Part model, mm, in its own coordinate system. Face numbers are marked on the shaded views. Give positions to 0.01 mm unless a question says otherwise; leave off trailing zeros. Order: outer loops, then holes, each group sorted by start corner. A loop starts at its lowest first (then second) coordinate and runs counter-clockwise, first axis right, second up. Notation, with made-up numbers: M 21,25 L 37,25 A13 ccw 37,49 Z; hole C -25.75,-4.5 d9. An arc over 180 degrees is marked long. Answer as a JSON object with one key per item and string values.
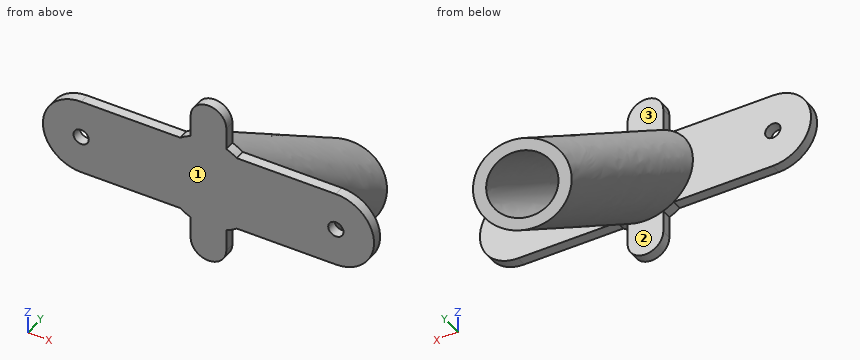
from build123d import *

# Parameters (mm, degrees)
CROQUIS1_R                 = 9.325
CROQUIS1_R_2               = 6.835
CROQUIS11_R                = 1.5
SALIENTE_EXTRUIR1_DEPTH    = 2
CORTAR_EXTRUIR2_DEPTH      = 69.96775808
CORTAR_EXTRUIR2_DEPTH_BACK = 69.96775808


with BuildPart() as part:
    # Barrer1: sweep along a path in Croquis6
    with BuildLine(Plane(origin=(0, 0, 0), x_dir=(0, 0, -1), z_dir=(1, 0, 0))) as barrer1_path:
        Line((9.345393917, 0), (40.892097916, 45.053362436))
    # Croquis1 → Barrer1 (sweep)
    with BuildSketch(Plane(origin=(0, 0, 0), x_dir=(1, 0, 0), z_dir=(0, 1, 0))):
        Circle(CROQUIS1_R)
        Circle(CROQUIS1_R_2, mode=Mode.SUBTRACT)
    sweep(path=barrer1_path.line)

    # Croquis11 → Saliente-Extruir1 (add)
    with BuildSketch(Plane.XZ):
        with BuildLine():
            Line((-25, 7.5), (-5.54126565, 7.5))
            ThreePointArc((-5.54126565, 7.5), (-4.556629397, 8.135892916), (-3.5, 8.643241579))
            Line((-3.5, 8.643241579), (-3.5, 13))
            ThreePointArc((-3.5, 13), (0, 16.5), (3.5, 13))
            Line((3.5, 13), (3.5, 8.643241579))
            ThreePointArc((3.5, 8.643241579), (4.556629397, 8.135892916), (5.54126565, 7.5))
            Line((5.54126565, 7.5), (25, 7.5))
            ThreePointArc((25, 7.5), (32.5, 0), (25, -7.5))
            Line((25, -7.5), (5.54126565, -7.5))
            ThreePointArc((5.54126565, -7.5), (4.556629397, -8.135892916), (3.5, -8.643241579))
            Line((3.5, -8.643241579), (3.5, -13))
            ThreePointArc((3.5, -13), (0, -16.5), (-3.5, -13))
            Line((-3.5, -13), (-3.5, -8.643241579))
            ThreePointArc((-3.5, -8.643241579), (-4.556629397, -8.135892916), (-5.54126565, -7.5))
            Line((-5.54126565, -7.5), (-25, -7.5))
            ThreePointArc((-25, -7.5), (-32.5, 0), (-25, 7.5))
        make_face()
        with Locations(Location((-25, 0, 0), (0, 0, 270))):
            Circle(CROQUIS11_R, mode=Mode.SUBTRACT)
        with Locations(Location((25, 0, 0), (0, 0, 270))):
            Circle(CROQUIS11_R, mode=Mode.SUBTRACT)
    extrude(amount=SALIENTE_EXTRUIR1_DEPTH)

    # Croquis13 → Cortar-Extruir2 (cut, two sides: drawn at the far end of the back side and taken through both)
    with BuildSketch(Plane(origin=(0, 0, 0), x_dir=(0, 0, -1), z_dir=(1, 0, 0)).offset(-CORTAR_EXTRUIR2_DEPTH_BACK)):
        Polygon((22.221703999, 45.053362436), (40.871703999, 31.994491848), (40.871703999, 45.053362436), align=None)
    extrude(amount=CORTAR_EXTRUIR2_DEPTH + CORTAR_EXTRUIR2_DEPTH_BACK, mode=Mode.SUBTRACT)


solid = part.part
1. Pin check, flat tips, straight feed: P1, Ø1, axis at y = -0.5, z = -10, coming from the +X side; P2, Ø6, axis at x = 12, z = 3.5, coming from the +Y side; P3, Ø2, axis at y = -1, z = 10.5, coming from the -X side; P4, Ø2.5, axis at x = 25, z = 0, coming from the -Y side. Stop position of each tip, or through.
Worked answers:
{"P1": "stops at x = 3.5", "P2": "stops at y = 0", "P3": "stops at x = -3.5", "P4": "passes through"}
2. Probe line 1 along X through (y, z) = (-1.3, 0); line 2 along X through (y, z) = (26, -18.5); line 3 along Y through (x, z) = (-25.5, 1.5). List the from-to ranges inside material, lowest first.
Worked answers:
{"line 1": "x = -32.5 to -26.5, -23.5 to 23.5, 26.5 to 32.5", "line 2": "x = -9.32 to -6.83, 6.83 to 9.32", "line 3": "y = -2 to 0"}
3. Two-plate mould, pull along Y, no slides. Class the marked faces 1, 2 and 3: +Y half, -Y half, draft (parallel to the pull), parting line (faces both ways), or undercut.
Worked answers:
{"face 1": "-Y half", "face 2": "undercut", "face 3": "+Y half"}
4. Cut at A-A on z = 0. State how many separate pieces and enclosed holes the cut face has, plus the area to 3 significant figures.
Worked answers:
{"separate pieces": "3", "enclosed holes": "1", "area": "208 mm^2"}
5. Cut at B-B on x = -11. Give the cut face in (y, z).
Worked answers:
{"outline": "M -2,-7.5 L 0,-7.5 L 0,7.5 L -2,7.5 Z"}
